from build123d import *

# Parameters (mm, degrees)
BOSS_EXTRUDE1_DEPTH      = 508
BOSS_EXTRUDE1_DEPTH_BACK = 254
SKETCH1_W                = 635
SKETCH1_H                = 635
SKETCH1_R                = 285.75


with BuildPart() as part:
    # Sketch1 → Boss-Extrude1 (new, two sides: drawn at the far end of the back side and taken through both)
    with BuildSketch(Plane(origin=(0, 0, 0), x_dir=(1, 0, 0), z_dir=(0, 1, 0)).offset(-BOSS_EXTRUDE1_DEPTH_BACK)):
        Rectangle(SKETCH1_W, SKETCH1_H)
        with Locations(Location((0, 0, 0), (0, 0, 270))):
            Circle(SKETCH1_R, mode=Mode.SUBTRACT)
    extrude(amount=BOSS_EXTRUDE1_DEPTH + BOSS_EXTRUDE1_DEPTH_BACK)


solid = part.part
The model under review builds one solid part; all positions refer to its coordinate system, in mm. Coordinates: 2 decimals unless noted, no trailing zeros. Loops run counter-clockwise (first coordinate to the right, second up) from the corner with the lowest first, then second, coordinate; pieces in that order, holes last.
(1) Consider section C-C, the plane y = 170.5. Give the boundary of the cut face in (x, z), plus the area to 3 significant figures.
Determined:
outline: (-317.5, -317.5) - (317.5, -317.5) - (317.5, 317.5) - (-317.5, 317.5) - close; hole circle Ø571.5 at (0, 0)
area: 147,000 mm2
(2) Draft analysis for pull direction X (two halves, no side actions). For faces 1 (the flat face through (-4, 122, 317.5)), 2 (the flat face through (317.5, 122, 4)), 3 (the flat face through (-317.5, 122, 4)), 4 (the cylindrical face through (85.832, 121.666, 272.555)), state which applies: +X half, -X half, draft (parallel to the pull), parting line (faces both ways), or undercut.
Determined:
face 1: draft
face 2: +X half
face 3: -X half
face 4: undercut
(3) Consider section A-A, the plane x = 0. Give the boundary of the cut face in (y, z).
Determined:
outline: (-254, -317.5) - (508, -317.5) - (508, -285.75) - (-254, -285.75) - close; (-254, 285.75) - (508, 285.75) - (508, 317.5) - (-254, 317.5) - close
(4) Consider section B-B, the plane z = 135.5. Give the boundary of the cut face in (x, y), plus the area to 3 significant figures.
Determined:
outline: (-317.5, -254) - (-251.58, -254) - (-251.58, 508) - (-317.5, 508) - close; (251.58, -254) - (317.5, -254) - (317.5, 508) - (251.58, 508) - close
area: 100,000 mm2
(5) Wall thickness on L1, parallel to X at y = 294, z = 0; L2, parallel to Z at x = 4, y = 252; L3, parallel to X at y = 185, z = 85: over which ranges is each line inside the solid? List them lowest first.
Determined:
L1: x = -317.5 to -285.75, 285.75 to 317.5
L2: z = -317.5 to -285.72, 285.72 to 317.5
L3: x = -317.5 to -272.82, 272.82 to 317.5
